Here's how the part is built. I have some questions about the finished solid (model axes, mm). A direction names the side the tool comes from. Coordinates: 2 decimals unless noted, no trailing zeros. Loops run counter-clockwise (first coordinate to the right, second up) from the corner with the lowest first, then second, coordinate; pieces in that order, holes last. Notation, with made-up numbers: (52.5, 32.25) -> (93.5, 32.25) arc R19 cw to (93.5, 62.25) -> close; hole circle Ø10 at (18, 6.5). An arc over 180 degrees is marked (long way). Answer as a JSON object with one key per item and string values. Group by question number.
1) I need wall thicknesses on probe 1 along X at (y, z) = (0, 14.3); probe 2 along X at (y, z) = (0, 5). Which ranges of each line are inside material? Lowest first, please. Write a range as [from, to].
2) I want a section at B-B (z = 9.5). Write out the boundary of the cut face in (x, y), then the cut area to 3 significant figures.
3) If we mould it in two halves opening along X, with no side actions, what happens to faces 1 (the flat face through (3.63, 6.16, 8.26)), 2 (the flat face through (-3.63, -6.16, 8.26)), 3 (the cylindrical face through (-3.27, 2.08, 14.64))? For each: +X half, -X half, draft (parallel to the pull), parting line (faces both ways), or undercut.
4) I'm going to push flat-ended pins straight in: pin 1 (1 mm diameter, centred on x = 0.5, z = 2.5, fed in from +Y); pin 2 (8 mm diameter, centred on x = -5, z = 13, fed in from +Y); pin 3 (8 mm diameter, centred on x = 2, z = 10.5, fed in from +Y); pin 4 (2 mm diameter, centred on y = -6, z = 4, fed in from -X). Where does each tip first touch, or does it pass through?
5) Which directions (+Z, -Z, +X, -X, +Y, -Y) give clear straight access to the entire face, cutting with the end or side of a thin tool? Please do faces 4 (the cylindrical face through (-0.31, -7.13, 1.69)), 5 (the flat face through (3.525, -6.221, 8.259)), 6 (the cylindrical face through (-0.31, -7.13, 14.21)).
```python
from build123d import *

# Parameters (mm, degrees)
BOSS_EXTRUDE1_DEPTH = 15.748
FILLET1_R           = 0.7874
CHAMFER1_SIZE       = 0.254
CHAMFER2_SIZE       = 0.127


with BuildPart() as part:
    # Sketch1 → Boss-Extrude1 (new body)
    with BuildSketch(Plane.XY):
        Polygon((0, 8.256224319), (-7.1501, 4.12811216), (-7.1501, -4.12811216), (0, -8.256224319), (7.1501, -4.12811216), (7.1501, 4.12811216), align=None)
    extrude(amount=BOSS_EXTRUDE1_DEPTH)

    # Sketch2 → Cut-Revolve1 (revolve, cut)
    with BuildSketch(Plane(origin=(0, 0, 0), x_dir=(0, 0, -1), z_dir=(1, 0, 0))):
        Polygon((-15.748, 9.375048639), (-15.748, 7.1374), (-13.4874, 7.1374), (-13.187611927, 8.256224319), (-3.474788073, 8.256224319), (-3.175, 7.1374), (0, 7.1374), (0, 9.375048639), align=None)
        with BuildLine():
            Line((-15.748, 3.8735), (-15.748, 0))
            Line((-15.748, 0), (0, 0))
            Line((0, 0), (0, 4.782916378))
            Line((0, 4.782916378), (-13.2588, 4.782916378))
            ThreePointArc((-13.2588, 4.782916378), (-13.438405122, 4.7085215), (-13.5128, 4.528916378))
            Line((-13.5128, 4.528916378), (-13.5128, 3.8735))
            Line((-13.5128, 3.8735), (-15.748, 3.8735))
        make_face()
    revolve(axis=Axis((0, 0, 0), (0, 0, 1)), mode=Mode.SUBTRACT)

    # Fillet1
    fillet1_edges = [part.edges().sort_by_distance(p)[0] for p in [
        (0, -7.1374, 15.748),
    ]]
    fillet(fillet1_edges, radius=FILLET1_R)

    # Chamfer1
    chamfer1_edges = [part.edges().sort_by_distance(p)[0] for p in [
        (0, -7.1374, 0),
    ]]
    chamfer(chamfer1_edges, length=CHAMFER1_SIZE)

    # Chamfer2
    chamfer2_edges = [part.edges().sort_by_distance(p)[0] for p in [
        (0, -3.8735, 15.748),
        (0, -3.8735, 13.5128),
    ]]
    chamfer(chamfer2_edges, length=CHAMFER2_SIZE)


solid = part.part
```
Determined:
{
 "1": {"probe 1": "[-7.14, -3.87], [3.87, 7.14]", "probe 2": "[-7.15, -4.78], [4.78, 7.15]"},
 "2": {"outline": "(-7.15, -4.13) -> (0, -8.26) -> (7.15, -4.13) -> (7.15, 4.13) -> (0, 8.26) -> (-7.15, 4.13) -> close; hole circle Ø9.57 at (0, 0)", "area": "105 mm^2"},
 "3": {"face 1": "+X half", "face 2": "-X half", "face 3": "undercut"},
 "4": {"pin 1": "y = 7.14", "pin 2": "y = 7.68", "pin 3": "y = 8.26", "pin 4": "x = -5.64"},
 "5": {"face 4": "-Z", "face 5": "+Z, -Z, +X, -Y", "face 6": "+Z"}
}
